Read the model definition and answer for the solid it produces. Units are mm, in the model's axes. Face numbers are marked on the shaded views. A direction names the side the tool comes from. Coordinates: 2 decimals unless noted, no trailing zeros. Write each loop counter-clockwise with the first axis right and the second up, starting at its lowest first coordinate (ties: lowest second). Pieces come first, ordered by that corner, then holes.
Item 1: Section C-C (z = 3.75) is taken. Give the vertices of the cut face in (x, y) (3 decimals), then the cut area to 3 significant figures.
Item 2: Section D-D (x = -1.5) is taken. Give the vertices of the cut face in (y, z).
Item 3: Determine the mould class of the marked faces 5, 6 and 7 for opening direction X: released by +X, released by -X, zero draft, split by the parting line, or undercut.
Item 4: Each of these flat-tipped pins is pushed along its axis until it touches: P1, Ø0.5, axis at x = 8.5, z = 4.5, coming from the -Y side; P2, Ø3, axis at y = -3, z = 2.5, coming from the +X side; P3, Ø1.6, axis at x = 6.5, z = 2, coming from the -Y side. Where does it stop, or does it pass through?
Item 5: A tool of negligible diameter and unlimited length cuts with its end or side. For the marked faces 1, 2, 3 and 4, from which of +Z, -Z, +X, -X, +Y, -Y can it reach the whole face along a straight path? Write none if from no direction.
Item 6: Straight lines are drawn through the part: probe 1 along Y at (x, z) = (8, 0.5); probe 2 along X at (y, z) = (-4.25, 3) (3 decimals); probe 3 along X at (y, z) = (5.75, 2.25) (3 decimals). For each, find the intervals that lie inside material, in ascending order.
Item 7: Section A-A (y = 7) is taken. Give the vertices of the cut face in (x, z) (3 decimals), then the cut area to 3 significant figures.
Item 8: Section B-B (x = 4.25) is taken. Give the vertices of the cut face in (y, z).
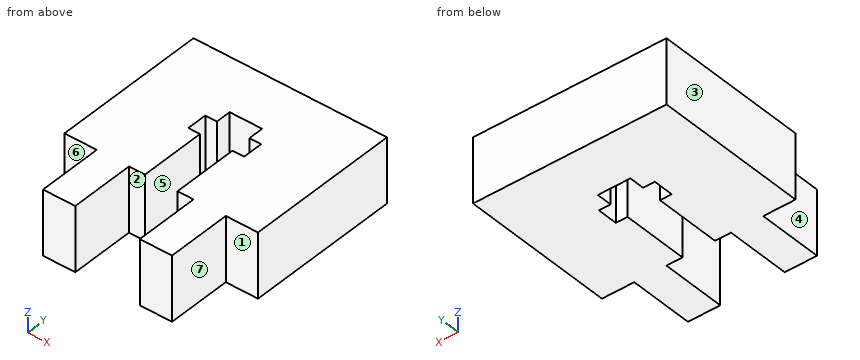
from build123d import *

# Parameters (mm, degrees)
BOSS_EXTRUDE1_DEPTH = 6.35
CUT_EXTRUDE3_DEPTH  = 7.35


with BuildPart() as part:
    # Sketch1 → Boss-Extrude1 (new body)
    with BuildSketch(Plane.XY):
        Polygon((-3.175, 15.24), (15.875, 15.24), (15.875, 0), (12.7, 0), (12.7, -6.35), (9.525, -6.35), (9.525, 0), (3.175, 0), (3.175, -6.35), (0, -6.35), (0, 0), (-3.175, 0), align=None)
    extrude(amount=BOSS_EXTRUDE1_DEPTH)

    # Sketch3 → Cut-Extrude3 (cut, through all)
    with BuildSketch(Plane.XY.offset(6.35)):
        Polygon((4.75, 0), (7.95, 0), (7.95, 6.5), (9.1, 6.5), (9.1, 8.5), (7.95, 8.5), (7.95, 10), (4.75, 10), (4.75, 8.5), (3.6, 8.5), (3.6, 6.5), (4.75, 6.5), align=None)
    extrude(amount=-CUT_EXTRUDE3_DEPTH, mode=Mode.SUBTRACT)


solid = part.part
Established:
1. outline: (-3.175, 0) - (0, 0) - (0, -6.35) - (3.175, -6.35) - (3.175, 0) - (4.75, 0) - (4.75, 6.5) - (3.6, 6.5) - (3.6, 8.5) - (4.75, 8.5) - (4.75, 10) - (7.95, 10) - (7.95, 8.5) - (9.1, 8.5) - (9.1, 6.5) - (7.95, 6.5) - (7.95, 0) - (9.525, 0) - (9.525, -6.35) - (12.7, -6.35) - (12.7, 0) - (15.875, 0) - (15.875, 15.24) - (-3.175, 15.24) - close
1. area: 294 mm2
2. outline: (0, 0) - (15.24, 0) - (15.24, 6.35) - (0, 6.35) - close
3. face 5: undercut
3. face 6: zero draft
3. face 7: released by +X
4. P1: stops at y = 0
4. P2: stops at x = 12.7
4. P3: stops at y = 10
5. face 1: +Z, -Z, +X, -Y
5. face 2: +Z, -Z, -Y
5. face 3: +Z, -Z, -X, +Y, -Y
5. face 4: +Z, -Z, -X, -Y
6. probe 1: y = 0 to 6.5, 8.5 to 15.24
6. probe 2: x = 0 to 3.175, 9.525 to 12.7
6. probe 3: x = -3.175 to 4.75, 7.95 to 15.875
7. outline: (-3.175, 0) - (3.6, 0) - (3.6, 6.35) - (-3.175, 6.35) - close; (9.1, 0) - (15.875, 0) - (15.875, 6.35) - (9.1, 6.35) - close
7. area: 86.0 mm2
8. outline: (0, 0) - (6.5, 0) - (6.5, 6.35) - (0, 6.35) - close; (8.5, 0) - (15.24, 0) - (15.24, 6.35) - (8.5, 6.35) - close
